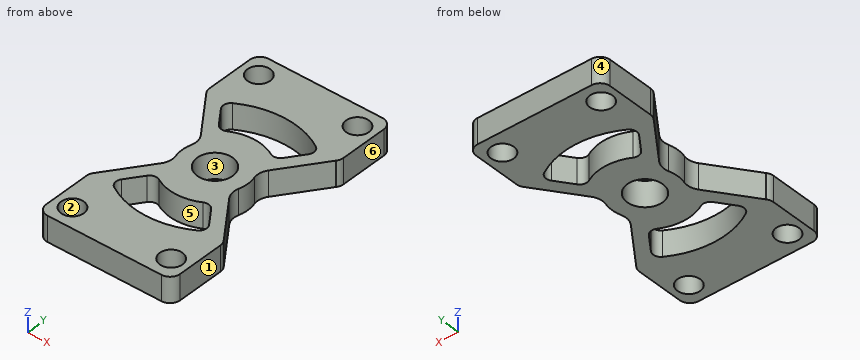
Autodesk Inventor part; units mm, degrees
ref_plane "YZ Plane" through (0, 0, 0) normal (1, 0, 0) x (0, 1, 0)
ref_plane "XZ Plane" through (0, 0, 0) normal (0, 1, 0) x (-1, 0, 0)
ref_plane "XY Plane" through (0, 0, 0) normal (0, 0, 1) x (1, 0, 0)
sketch "Sketch1" plane through (0, 0, 0) normal (0, 0, 1) x (1, 0, 0)
  circle A0 centre (9.7751, -3.2289) radius 1.621
  circle A1 centre (-9.7751, -3.2289) radius 1.621
  line L0 (-11.2751, -7.2289) -> (11.2751, -7.2289)
  line L1 (13.2751, -5.2289) -> (13.2751, 4.1213)
  line L2 (12.8932, 5.2968) -> (12.7957, 5.4309)
  line L3 (-12.7957, 5.4309) -> (-12.8932, 5.2968)
  line L4 (-13.2751, 4.1213) -> (-13.2751, -5.2289)
  circle A2 centre (-9.7751, 39.9572) radius 1.621
  circle A3 centre (9.7751, 39.9572) radius 1.621
  line L5 (11.2751, 43.9572) -> (-11.2751, 43.9572)
  line L6 (-13.2751, 41.9572) -> (-13.2751, 32.607)
  line L7 (-12.8932, 31.4315) -> (-12.7957, 31.2974)
  line L8 (12.7957, 31.2974) -> (12.8932, 31.4315)
  line L9 (13.2751, 32.607) -> (13.2751, 41.9572)
  line L10 (13.2751, -7.2289) -> (-13.2751, -7.2289)
  line L11 (-13.2751, -7.2289) -> (-13.2751, 43.9572)
  line L12 (-13.2751, 43.9572) -> (13.2751, 43.9572)
  line L13 (13.2751, 43.9572) -> (13.2751, -7.2289)
  circle A4 centre (0, 18.3641) radius 3.5
  circle A5 centre (0, 18.3641) radius 6.5
  line L14 (13.2751, 31.9572) -> (5.6866, 21.5125)
  line L15 (13.2751, 4.7711) -> (5.6866, 15.2158)
  line L16 (-13.2751, 4.7711) -> (-5.6866, 15.2158)
  line L17 (-13.2751, 31.9572) -> (-5.6866, 21.5125)
  arc A6 (-11.4894, 7.2289) -> (11.4894, 7.2289) centre (0, 18.3641) ccw
  arc A7 (11.4894, 29.4994) -> (-11.4894, 29.4994) centre (0, 18.3641) ccw
  line L18 (5.6866, 15.2158) -> (11.4894, 7.2289)
  line L19 (-5.6866, 15.2158) -> (-11.4894, 7.2289)
  arc A8 (-5.6866, 15.2158) -> (5.6866, 15.2158) centre (0, 18.3641) ccw
  line L20 (5.4903, 11.2327) -> (9.6057, 5.5684)
  arc A9 (-5.4903, 11.2327) -> (5.4903, 11.2327) centre (0, 18.3641) ccw
  line L21 (-9.6057, 5.5684) -> (-5.4903, 11.2327)
  line L22 (0, 18.3641) -> (-13.2751, 18.3641) construction
  circle A10 centre (0, 18.3641) radius 6.5 construction
  arc A11 (5.6866, 21.5125) -> (-5.6866, 21.5125) centre (0, 18.3641) ccw
  line L23 (5.4903, 25.4955) -> (9.6057, 31.1599)
  arc A12 (5.4903, 25.4955) -> (-5.4903, 25.4955) centre (0, 18.3641) ccw
  line L24 (-9.6057, 31.1599) -> (-4.02, 23.4719)
  arc A13 (-13.2751, 32.607) -> (-12.8932, 31.4315) centre (-11.2751, 32.607) ccw
  arc A14 (-12.7957, 31.2974) -> (-12.6739, 31.1458) centre (-11.1777, 32.473) ccw
  arc A15 (12.6739, 31.1458) -> (-12.6739, 31.1458) centre (0, 18.3641) ccw
  arc A16 (12.6739, 31.1458) -> (12.7957, 31.2974) centre (11.1777, 32.473) ccw
  arc A17 (12.8932, 31.4315) -> (13.2751, 32.607) centre (11.2751, 32.607) ccw
  arc A18 (13.2751, 41.9572) -> (11.2751, 43.9572) centre (11.2751, 41.9572) ccw
  arc A19 (-11.2751, 43.9572) -> (-13.2751, 41.9572) centre (-11.2751, 41.9572) ccw
  arc A20 (13.2751, 4.1213) -> (12.8932, 5.2968) centre (11.2751, 4.1213) ccw
  arc A21 (12.7957, 5.4309) -> (12.6739, 5.5825) centre (11.1777, 4.2553) ccw
  arc A22 (-12.6739, 5.5825) -> (12.6739, 5.5825) centre (0, 18.3641) ccw
  arc A23 (-12.6739, 5.5825) -> (-12.7957, 5.4309) centre (-11.1777, 4.2553) ccw
  arc A24 (-12.8932, 5.2968) -> (-13.2751, 4.1213) centre (-11.2751, 4.1213) ccw
  arc A25 (-13.2751, -5.2289) -> (-11.2751, -7.2289) centre (-11.2751, -5.2289) ccw
  arc A26 (11.2751, -7.2289) -> (13.2751, -5.2289) centre (11.2751, -5.2289) ccw
  point P0 (0, 0)
  point P1 (8.136, 7.5912)
  point P2 (-8.136, 7.5912)
  point P3 (8.136, 29.1371)
  point P4 (-8.136, 29.1371)
  dimension "d0" = 7
  dimension "d1" = 13
  dimension "d4" = 2.5
  dimension "d5" = 2.5
  dimension "d6" = 2.5
extrude "Extrusion1" add sketch "Sketch1" along normal blind 5 contours A25 L4 A24 L3 A23 A22 A21 L2 A20 L1 A26 L0 | L16 A6 L15 A21 A22 A23 | L6 A19 L5 A18 L9 A17 L8 A16 A15 A14 L7 A13 | L16 A5 L15 A6 L20 A9 L21 | A14 A15 A16 L14 A7 L17 | A5 | A7 L24 A5 L17 | L14 A5 L24 A12 L23 A7
fillet "Fillet1" radius 3.175 4 edges at (5.6866, 15.2158, 2.5) (5.6866, 21.5125, 2.5) (-5.6866, 15.2158, 2.5) (-5.6866, 21.5125, 2.5)
sketch "Sketch2" plane through (0, 0, 5) normal (0, 0, 1) x (1, 0, 0)
  circle A0 centre (9.7751, -3.2289) radius 1.621
  circle A1 centre (-9.7751, -3.2289) radius 1.621
  circle A2 centre (9.7751, 39.9572) radius 1.621
  circle A3 centre (-9.7751, 39.9572) radius 1.621
  circle A4 centre (9.7751, -3.2289) radius 1.621
  circle A5 centre (-9.7751, -3.2289) radius 1.621
  point P0 (0, 0)
hole "Hole1" at (9.7751, -3.2289, 5) at (-9.7751, -3.2289, 5) at (-9.7751, 39.9572, 5) at (9.7751, 39.9572, 5) direction (0, 0, -1) diameter 4.4958 end through all
fillet "Fillet2" radius 1.524 8 edges at (-9.6057, 31.1599, 2.5) (-5.4903, 25.4955, 2.5) (5.4903, 25.4955, 2.5) (9.6057, 31.1599, 2.5) (-9.6057, 5.5684, 2.5) (-5.4903, 11.2327, 2.5) (5.4903, 11.2327, 2.5) (9.6057, 5.5684, 2.5)
properties part number "2104_Tx_CoilBackPlate_V1"
Geometry: final body of the model. Coordinates: model frame, mm. Face numbers are marked on the shaded views. A direction names the side the tool comes from. Coordinates: 2 decimals unless noted, no trailing zeros. Write each loop counter-clockwise with the first axis right and the second up, starting at its lowest first coordinate (ties: lowest second). Pieces come first, ordered by that corner, then holes. Notation, with made-up numbers: (78, -12.5) - (90, -12.5) arc R8 ccw to (90, 2.5) - close; hole circle Ø5 at (-14.5, 78.5). An arc over 180 degrees is marked (long way). Return JSON: item names as keys, results as strings.
Item 1: Pull-direction query (X, two-part tool) for the marked faces 1, 2, 3 and 4; classes: +X half, -X half, draft (parallel to the pull), parting line (faces both ways), or undercut.
Completed:
{"face 1": "+X half", "face 2": "undercut", "face 3": "undercut", "face 4": "-X half"}
Item 2: Pin query (flat end, axial travel): pin 1 Ø1.5 at (x, y) = (7.5, 22.5) entering from -Z. Return the tip coordinate at first contact, or that it passes through.
Completed:
{"pin 1": "passes through"}
Item 3: Section query C-C (y = 13). Output: boundary loops of the cut face in (x, z), and give its area (3 significant figures).
Completed:
{"outline": "(-7.3, 0) - (7.3, 0) - (7.3, 5) - (-7.3, 5) - close", "area": "73.0 mm2"}
Item 4: Section query B-B (z = 0.65). Count the separate pieces of the cut face and the enclosed holes in it, and give its area (3 significant figures).
Completed:
{"separate pieces": "1", "enclosed holes": "7", "area": "785 mm2"}
Item 5: Reachability of the marked faces 5 and 6 from +Z, -Z, +X, -X, +Y, -Y: full face, straight path, thin tool, end or side. Return the list, or none.
Completed:
{"face 5": "+Z, -Z", "face 6": "+Z, -Z, +X, +Y, -Y"}
Item 6: Section query A-A (x = 0). Output: boundary loops of the cut face in (y, z), and give its area (3 significant figures).
Completed:
{"outline": "(-7.23, 0) - (2.36, 0) - (2.36, 5) - (-7.23, 5) - close; (9.36, 0) - (14.86, 0) - (14.86, 5) - (9.36, 5) - close; (21.86, 0) - (27.36, 0) - (27.36, 5) - (21.86, 5) - close; (34.36, 0) - (43.96, 0) - (43.96, 5) - (34.36, 5) - close", "area": "151 mm2"}
Item 7: Line query: L1, parallel to X at y = 40, z = 1.55; L2, parallel to Y at x = 0, z = 1.4; L3, parallel to X at y = 18.5, z = 3.85. Output: solid intervals per line, ascending.
Completed:
{"L1": "x = -13.28 to -12.02, -7.53 to 7.53, 12.02 to 13.28", "L2": "y = -7.23 to 2.36, 9.36 to 14.86, 21.86 to 27.36, 34.36 to 43.96", "L3": "x = -6.5 to -3.5, 3.5 to 6.5"}
